from build123d import *

# Parameters (mm, degrees)
SKETCH_1_W          = 250
SKETCH_1_H          = 300
EXTRUDE_1_DEPTH     = 300
SKETCH_2_W          = 230
SKETCH_2_H          = 280
CUT_EXTRUDE_1_DEPTH = 290
SKETCH_3_W          = 280
SKETCH_3_H          = 360
EXTRUDE_2_DEPTH     = 10
CUT_EXTRUDE_2_DEPTH = 10


with BuildPart() as part:
    # 草图1 → 凸台-拉伸1 (new body)
    with BuildSketch(Plane.XY):
        with Locations((125, 150)):
            Rectangle(SKETCH_1_W, SKETCH_1_H)
    extrude(amount=EXTRUDE_1_DEPTH)

    # 草图2 → 切除-拉伸1 (cut)
    with BuildSketch(Plane.XY.offset(300)):
        with Locations((125, 150)):
            Rectangle(SKETCH_2_W, SKETCH_2_H)
    extrude(amount=-CUT_EXTRUDE_1_DEPTH, mode=Mode.SUBTRACT)

    # 草图3 → 凸台-拉伸2 (add)
    with BuildSketch(Plane.XZ):
        with Locations((125, 150)):
            Rectangle(SKETCH_3_W, SKETCH_3_H)
    extrude(amount=EXTRUDE_2_DEPTH)

    # 草图4 → 切除-拉伸2 (cut)
    with BuildSketch(Plane.XZ.offset(10)):
        with BuildLine():
            Line((92.011234141, 284.219295629), (173.345605139, 284.219295629))
            ThreePointArc((173.345605139, 284.219295629), (187.564900768, 270), (173.345605139, 255.780704371))
            Line((173.345605139, 255.780704371), (92.011234141, 255.780704371))
            ThreePointArc((92.011234141, 255.780704371), (77.791938512, 270), (92.011234141, 284.219295629))
        make_face()
    extrude(amount=-CUT_EXTRUDE_2_DEPTH, mode=Mode.SUBTRACT)


solid = part.part
The model under review builds one solid part; all positions refer to its coordinate system, in mm. A direction names the side the tool comes from. Give positions to 0.01 mm unless a question says otherwise; leave off trailing zeros. Order: outer loops, then holes, each group sorted by start corner. A loop starts at its lowest first (then second) coordinate and runs counter-clockwise, first axis right, second up. Notation, with made-up numbers: M -26.75,37.25 L 5.25,37.25 A6 cw 5.25,43.25 Z; hole C -11.5,84.5 d5. An arc over 180 degrees is marked long. Answer in a Markdown table with one row per item. Add a question column.
1. Mouldability with a two-part tool opening along Y and no side actions: class faces 1 (the flat face through (4, 151, 300)), 2 (the flat face through (133, 0, 270)), 3 (the flat face through (10, 148, 157)) as released by +Y, released by -Y, zero draft, split by the parting line, or undercut.
2. Machinability: for faces 4 (the flat face through (123, 10, 157)), 5 (the flat face through (132, -5, 284.219)), 6 (the flat face through (0, 148, 148)), 7 (the flat face through (123, 152, 0)), which of the approach directions +Z, -Z, +X, -X, +Y, -Y give a long, thin tool a straight path to every point of the face, cutting with its end or side? Answer none if there is none.
3. Add section D-D on z = 270. State the section outline as (x, y) points.
4. Add section B-B on y = 156. State the section outline as (x, z) points.
5. To check wall thickness, follow line 1 along X through (y, z) = (83, 54.5); line 2 along Y through (x, z) = (170.5, 229); line 3 along Y through (x, z) = (85, 276). State the ranges of each line that lie inside material, in increasing order.
6. For pin 1 Ø6 at (y, z) = (74.5, 71) entering from +X; pin 2 Ø2 at (x, y) = (22.5, 202.5) entering from +Z; pin 3 Ø10 at (y, z) = (155.5, 253) entering from -X, all flat-tipped, find the tip position at first contact; note any pin that passes through.
7. Add section A-A on z = 107. State the section outline as (x, y) points.
8. Add section C-C on x = 72. State the section outline as (y, z) points, plus the area to 3 significant figures.
The answers:
| question | item | result |
|---|---|---|
| 1 | face 1 | zero draft |
| 1 | face 2 | released by -Y |
| 1 | face 3 | undercut |
| 2 | face 4 | +Z |
| 2 | face 5 | -Y |
| 2 | face 6 | +Z, -Z, -X, +Y |
| 2 | face 7 | -Z, +X, -X, +Y |
| 3 | outline | M -15,-10 L 77.79,-10 L 77.79,0 L 187.56,0 L 187.56,-10 L 265,-10 L 265,0 L 250,0 L 250,300 L 0,300 L 0,0 L -15,0 Z; hole M 10,10 L 240,10 L 240,290 L 10,290 Z |
| 4 | outline | M 0,0 L 250,0 L 250,300 L 240,300 L 240,10 L 10,10 L 10,300 L 0,300 Z |
| 5 | line 1 | 0 to 10, 240 to 250 |
| 5 | line 2 | -10 to 10, 290 to 300 |
| 5 | line 3 | 0 to 10, 290 to 300 |
| 6 | pin 1 | x = 250 |
| 6 | pin 2 | z = 10 |
| 6 | pin 3 | x = 0 |
| 7 | outline | M -15,-10 L 265,-10 L 265,0 L 250,0 L 250,300 L 0,300 L 0,0 L -15,0 Z; hole M 10,10 L 240,10 L 240,290 L 10,290 Z |
| 8 | outline | M -10,-30 L 0,-30 L 0,0 L 300,0 L 300,300 L 290,300 L 290,10 L 10,10 L 10,300 L 0,300 L 0,330 L -10,330 Z |
| 8 | area | 12,400 mm2 |
